from build123d import *

# Parameters (mm, degrees)
F3_W         = 27
F3_H         = 27
F4_DEPTH     = 30
F5_T1_DEPTH  = 662
F5_T3_DEPTH  = 392
F5_T5_DEPTH  = 350
F5_T10_DEPTH = 433
F5_T15_DEPTH = 703
F5_T17_DEPTH = 402
F5_T19_DEPTH = 672
F5_T21_DEPTH = 710
F5_T23_DEPTH = 440
F5_T25_DEPTH = 346
F5_T27_DEPTH = 390
F5_T29_DEPTH = 660
F5_T32_ANGLE = 90
F5_T33_DEPTH = 393
F5_T35_DEPTH = 663
F5_T38_ANGLE = 90
F5_T40_ANGLE = 90


# Not quite as in the source:
# - a fillet or chamfer that OpenCascade refuses, or shapes differently, is made with other operations: its cross-section is extruded or revolved along the edge and cut away or added


with BuildPart() as f2:
    # F2: sweep along a path in F1
    with BuildLine(Plane.XY) as f2_path:
        Line((0, 0), (0, 390))
        Line((0, 390), (-660, 390))
    # F0 (on Front) → F2 (sweep)
    with BuildSketch(Plane.XZ):
        Polygon((38, -2), (38, -25), (40, -25), (40, 0), (0, 0), (0, -350), (27, -350), (27, -376), (29, -376), (29, -348), (2, -348), (2, -2), align=None)
    sweep(path=f2_path.line, transition=Transition.RIGHT)

    # F3 (on face) → F4 (cut)
    with BuildSketch(Plane.XY.offset(-348)):
        with Locations((15.5, 405.5)):
            Rectangle(F3_W, F3_H)
    extrude(amount=-F4_DEPTH, mode=Mode.SUBTRACT)

    # F5: fillet of radius 2 on 16 edges, made by hand

    # F5_s2 → F5_t1 (join)
    with BuildSketch(Plane.YZ.offset(-660)):
        with BuildLine():
            ThreePointArc((415, -350), (416.4142135624, -350.5857864376), (417, -352))
            Line((417, -352), (417, -350))
            Line((417, -350), (415, -350))
        make_face()
    extrude(amount=F5_T1_DEPTH)

    # F5_s4 → F5_t3 (join)
    with BuildSketch(Plane.XZ.offset(-392)):
        with BuildLine():
            ThreePointArc((25, -350), (26.4142135624, -350.5857864376), (27, -352))
            Line((27, -352), (27, -350))
            Line((27, -350), (25, -350))
        make_face()
    extrude(amount=F5_T3_DEPTH)

    # F5_s6 → F5_t5 (join)
    with BuildSketch(Plane.XY.offset(-350)):
        with BuildLine():
            ThreePointArc((0, 388), (-0.5857864376, 389.4142135624), (-2, 390))
            Line((-2, 390), (0, 390))
            Line((0, 390), (0, 388))
        make_face()
    extrude(amount=F5_T5_DEPTH)


with BuildPart() as f5_tool8:
    # F5_s9 → F5_t10 (new body)
    with BuildSketch(Plane.XZ):
        with BuildLine():
            ThreePointArc((38, -4), (37.4142135624, -2.5857864376), (36, -2))
            Line((36, -2), (38, -2))
            Line((38, -2), (38, -4))
        make_face()
    extrude(amount=-F5_T10_DEPTH)

    split(bisect_by=Plane.XZ.offset(-430), keep=Keep.TOP)


with BuildPart() as f2_1:
    add(f2.part)

    # F5_t7: union F5_tool8
    add(f5_tool8.part)


with BuildPart() as f5_tool13:
    # F5_s14 → F5_t15 (new body)
    with BuildSketch(Plane.YZ.offset(43)):
        with BuildLine():
            ThreePointArc((426, -2), (427.4142135624, -2.5857864376), (428, -4))
            Line((428, -4), (428, -2))
            Line((428, -2), (426, -2))
        make_face()
    extrude(amount=-F5_T15_DEPTH)

    split(bisect_by=Plane.YZ.offset(40), keep=Keep.BOTTOM)


with BuildPart() as f2_2:
    add(f2_1.part)

    # F5_t12: union F5_tool13
    add(f5_tool13.part)

    # F5_s18 → F5_t17 (cut)
    with BuildSketch(Plane.XZ.offset(-397)):
        with BuildLine():
            ThreePointArc((29, -350), (28.4142135624, -348.5857864376), (27, -348))
            Line((27, -348), (29, -348))
            Line((29, -348), (29, -350))
        make_face()
    extrude(amount=F5_T17_DEPTH, mode=Mode.SUBTRACT)

    # F5_s20 → F5_t19 (cut)
    with BuildSketch(Plane.YZ.offset(-665)):
        with BuildLine():
            ThreePointArc((419, -350), (418.4142135624, -348.5857864376), (417, -348))
            Line((417, -348), (419, -348))
            Line((419, -348), (419, -350))
        make_face()
    extrude(amount=F5_T19_DEPTH, mode=Mode.SUBTRACT)

    # F5_s22 → F5_t21 (cut)
    with BuildSketch(Plane.YZ.offset(-665)):
        with BuildLine():
            ThreePointArc((430, -2), (429.4142135624, -0.5857864376), (428, 0))
            Line((428, 0), (430, 0))
            Line((430, 0), (430, -2))
        make_face()
    extrude(amount=F5_T21_DEPTH, mode=Mode.SUBTRACT)

    # F5_s24 → F5_t23 (cut)
    with BuildSketch(Plane.XZ.offset(-435)):
        with BuildLine():
            ThreePointArc((40, -2), (39.4142135624, -0.5857864376), (38, 0))
            Line((38, 0), (40, 0))
            Line((40, 0), (40, -2))
        make_face()
    extrude(amount=F5_T23_DEPTH, mode=Mode.SUBTRACT)

    # F5_s26 → F5_t25 (cut)
    with BuildSketch(Plane.XY.offset(-348)):
        with BuildLine():
            ThreePointArc((2, 390), (1.4142135624, 391.4142135624), (0, 392))
            Line((0, 392), (2, 392))
            Line((2, 392), (2, 390))
        make_face()
    extrude(amount=F5_T25_DEPTH, mode=Mode.SUBTRACT)

    # F5_s28 → F5_t27 (join)
    with BuildSketch(Plane.XZ.offset(-390)):
        with BuildLine():
            ThreePointArc((4, -2), (2.5857864376, -2.5857864376), (2, -4))
            Line((2, -4), (2, -2))
            Line((2, -2), (4, -2))
        make_face()
    extrude(amount=F5_T27_DEPTH)

    # F5_s30 → F5_t29 (join)
    with BuildSketch(Plane.YZ.offset(-660)):
        with BuildLine():
            ThreePointArc((394, -2), (392.5857864376, -2.5857864376), (392, -4))
            Line((392, -4), (392, -2))
            Line((392, -2), (394, -2))
        make_face()
    extrude(amount=F5_T29_DEPTH)

    # F5_s31 → F5_t32 (revolve)
    with BuildSketch(Plane.XZ.offset(-390)):
        with BuildLine():
            ThreePointArc((4, -2), (2.5857864376, -2.5857864376), (2, -4))
            Line((2, -4), (2, -2))
            Line((2, -2), (4, -2))
        make_face()
    revolve(axis=Axis((0, 390, -2), (0, 0, 1)), revolution_arc=F5_T32_ANGLE)

    # F5_s34 → F5_t33 (cut)
    with BuildSketch(Plane.XZ.offset(-388)):
        with BuildLine():
            ThreePointArc((2, -350), (0.5857864376, -349.4142135624), (0, -348))
            Line((0, -348), (0, -350))
            Line((0, -350), (2, -350))
        make_face()
        with BuildLine():
            ThreePointArc((0, -2), (0.5857864376, -0.5857864376), (2, 0))
            Line((2, 0), (0, 0))
            Line((0, 0), (0, -2))
        make_face()
    extrude(amount=F5_T33_DEPTH, mode=Mode.SUBTRACT)

    # F5_s36 → F5_t35 (cut)
    with BuildSketch(Plane.YZ.offset(-665)):
        with BuildLine():
            ThreePointArc((392, -350), (390.5857864376, -349.4142135624), (390, -348))
            Line((390, -348), (390, -350))
            Line((390, -350), (392, -350))
        make_face()
        with BuildLine():
            ThreePointArc((392, 0), (390.5857864376, -0.5857864376), (390, -2))
            Line((390, -2), (390, 0))
            Line((390, 0), (392, 0))
        make_face()
    extrude(amount=F5_T35_DEPTH, mode=Mode.SUBTRACT)

    # F5_s37 → F5_t38 (revolve, cut)
    with BuildSketch(Plane.XZ.offset(-388)):
        with BuildLine():
            ThreePointArc((2, 0), (0.5857864376, -0.5857864376), (0, -2))
            Line((0, -2), (0, 0))
            Line((0, 0), (2, 0))
        make_face()
    revolve(axis=Axis((-2, 388, 0), (0, 0, 1)), revolution_arc=F5_T38_ANGLE, mode=Mode.SUBTRACT)

    # F5_s39 → F5_t40 (revolve, cut)
    with BuildSketch(Plane.XZ.offset(-388)):
        with BuildLine():
            ThreePointArc((2, -350), (0.5857864376, -349.4142135624), (0, -348))
            Line((0, -348), (0, -350))
            Line((0, -350), (2, -350))
        make_face()
    revolve(axis=Axis((-2, 388, -350), (0, 0, 1)), revolution_arc=F5_T40_ANGLE, mode=Mode.SUBTRACT)


solid = f2_2.part
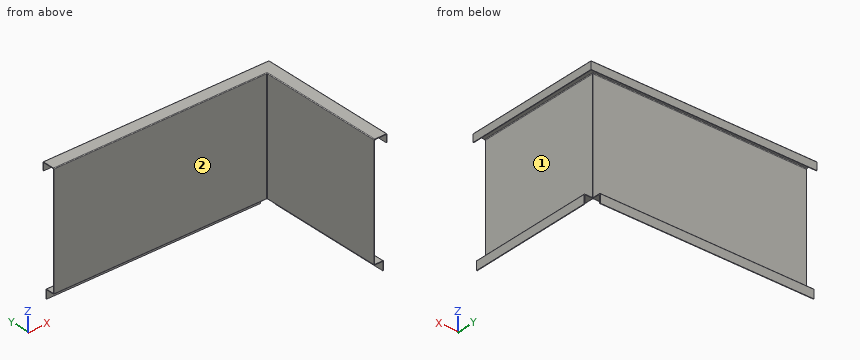
Model file for the job. Use its own axes, mm. Face numbers are marked on the shaded views. Give positions to 0.01 mm unless a question says otherwise; leave off trailing zeros. Loops run counter-clockwise (first coordinate to the right, second up) from the corner with the lowest first, then second, coordinate; pieces in that order, holes last. Notation, with made-up numbers: (33.5, 33.5) - (85.5, 33.5) arc R13 cw to (85.5, 42.5) - close; hole circle Ø10 at (-38, -10.5). An arc over 180 degrees is marked (long way). Use one line per item in the form item = value.
(1) Pull direction Z, two halves, no side cores. Call the marked faces 1 and 2: pulls with the +Z half, pulls with the -Z half, needs draft (parallel to the pull), parting line crosses it, or undercut.
Determined:
face_1 = undercut
face_2 = needs draft
(2) Cut at B-B (y = 197.5). Give the cut face in (x, z), then the cut area to 3 significant figures.
Determined:
outline = (0, -348) arc R2 ccw to (2, -350) - (25, -350) arc R2 cw to (27, -352) - (27, -376) - (29, -376) - (29, -350) arc R2 ccw to (27, -348) - (2, -348) - (2, -4) arc R2 cw to (4, -2) - (36, -2) arc R2 cw to (38, -4) - (38, -25) - (40, -25) - (40, -2) arc R2 ccw to (38, 0) - (2, 0) arc R2 ccw to (0, -2) - close
area = 927 mm^2
(3) Cut at A-A (x = -103). Give the cut face in (y, z), then the cut area to 3 significant figures.
Determined:
outline = (390, -348) arc R2 ccw to (392, -350) - (415, -350) arc R2 cw to (417, -352) - (417, -376) - (419, -376) - (419, -350) arc R2 ccw to (417, -348) - (392, -348) - (392, -4) arc R2 cw to (394, -2) - (426, -2) arc R2 cw to (428, -4) - (428, -25) - (430, -25) - (430, -2) arc R2 ccw to (428, 0) - (392, 0) arc R2 ccw to (390, -2) - close
area = 927 mm^2
(4) Drop flat-ended pins along their axis: P1, Ø6.5, axis at x = -419, z = -18.5, coming from the -Y side; P2, Ø23, axis at y = 210.5, z = -12.5, coming from the -X side; P3, Ø2, axis at x = -299, z = -248, coming from the +Y side. Give the stop position or say it passes through.
Determined:
P1 = 390
P2 = 0
P3 = 392
(5) Cut at C-C (z = -212.5). Give the cut face in (x, y).
Determined:
outline = (-660, 390) - (-2, 390) arc R2 cw to (0, 388) - (0, 0) - (2, 0) - (2, 390) arc R2 ccw to (0, 392) - (-660, 392) - close
(6) Drill centre lines: L1, parallel to Z at x = -337.5, y = 411; L2, parallel to X at y = 32, z = -162; L3, parallel to Y at x = -374.5, z = -171. Where is each one in solid material? Low to high.
Determined:
L1 = -350 to -348, -2 to 0
L2 = 0 to 2
L3 = 390 to 392
